Could you check a few things on this drawing? It's one solid part, dimensions in mm from its lowest x, y, z. A direction names the side the tool comes from. Coordinates: 2 decimals unless noted, no trailing zeros. Write each loop counter-clockwise with the first axis right and the second up, starting at its lowest first coordinate (ties: lowest second). Pieces come first, ordered by that corner, then holes.
Item 1: I want a section at B-B (x = 120). Please give me the cut outline in (y, z), and give its area (3 significant figures).
Item 2: I want a section at A-A (z = 17.5). Please give me the cut outline in (x, y).
Item 3: I want a section at C-C (y = 59). Please give me the cut outline in (x, z).
Item 4: I'm going to push flat-ended pins straight in: P1, Ø4, axis at y = 58, z = 188.5, coming from the +X side; P2, Ø22, axis at x = 218, y = 55.5, coming from the +Z side; P3, Ø6, axis at y = 57.5, z = 162.5, coming from the +X side. Where does each tip first touch, or does it pass through?
Item 5: Please list where these lines run through material, in increasing order: line 1 (Z direction, x = 120, y = 73); line 2 (Z direction, x = 114, y = 69.5); line 3 (Z direction, x = 29, y = 29.5).
Item 6: If we mould it in two halves opening along Z, with no side actions, what happens to the marked faces 1, 2 and 3? For each: pulls with the +Z half, pulls with the -Z half, needs draft (parallel to the pull), parting line crosses it, or undercut.
Item 7: For the marked faces 4 and 5, which set-ups out of +Z, -Z, +X, -X, +Y, -Y let a thin tool reach every point of the face, with its end or its side?
Item 8: I want a section at D-D (z = 146). Please give me the cut outline in (x, y).
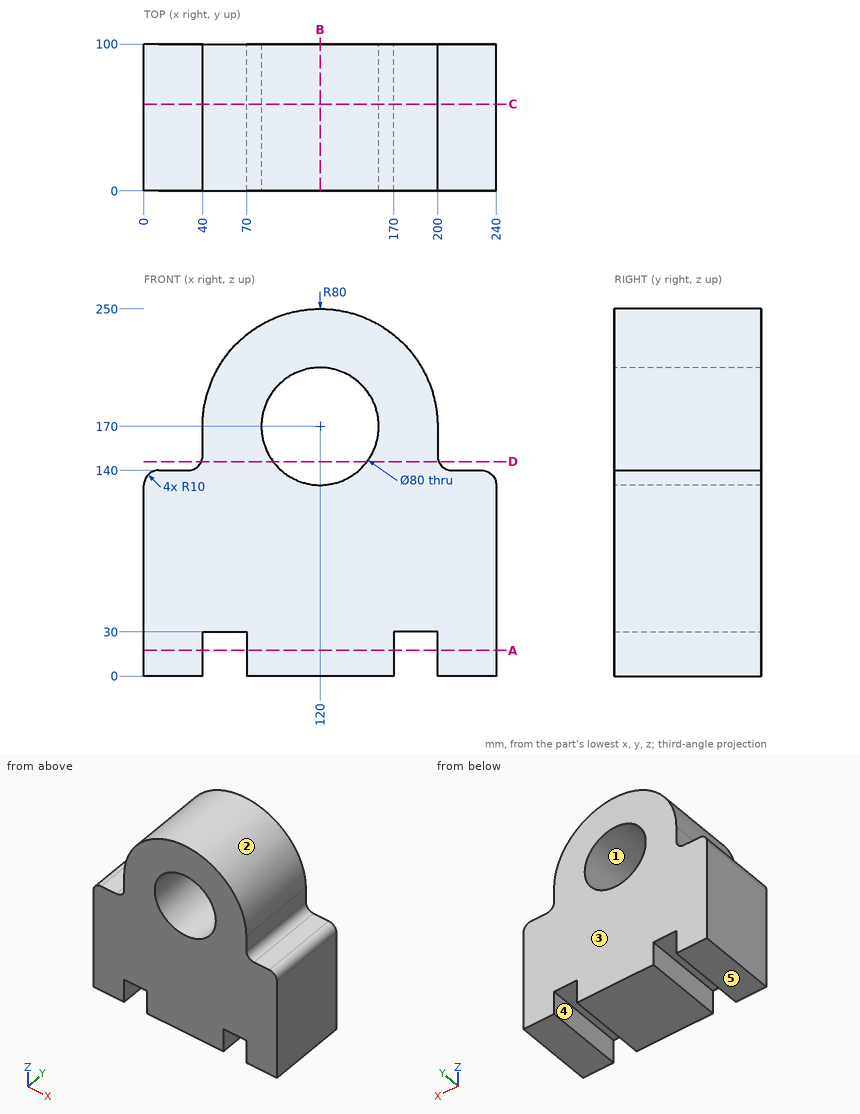
Answer:
1. outline: (0, 0) - (100, 0) - (100, 130) - (0, 130) - close; (0, 210) - (100, 210) - (100, 250) - (0, 250) - close
1. area: 17,000 mm2
2. outline: (0, 0) - (40, 0) - (40, 100) - (0, 100) - close; (70, 0) - (170, 0) - (170, 100) - (70, 100) - close; (200, 0) - (240, 0) - (240, 100) - (200, 100) - close
3. outline: (0, 0) - (40, 0) - (40, 30) - (70, 30) - (70, 0) - (170, 0) - (170, 30) - (200, 30) - (200, 0) - (240, 0) - (240, 130) arc R10 ccw to (230, 140) - (210, 140) arc R10 cw to (200, 150) - (200, 170) arc R80 ccw to (40, 170) - (40, 150) arc R10 cw to (30, 140) - (10, 140) arc R10 ccw to (0, 130) - close; hole circle Ø80 at (120, 170)
4. P1: stops at x = 198.28
4. P2: stops at z = 140.46
4. P3: stops at x = 200
5. line 1: z = 0 to 130, 210 to 250
5. line 2: z = 0 to 130.45, 209.55 to 249.77
5. line 3: z = 0 to 140
6. face 1: undercut
6. face 2: pulls with the +Z half
6. face 3: needs draft
7. face 4: -Z, +Y, -Y
7. face 5: -Z, +X, -X, +Y, -Y
8. outline: (39.17, 0) - (88, 0) - (88, 100) - (39.17, 100) - close; (152, 0) - (200.83, 0) - (200.83, 100) - (152, 100) - close
